```python
from build123d import *

# Parameters (mm, degrees)
SKETCH1_R           = 50.8
BOSS_EXTRUDE1_DEPTH = 228.6
SKETCH2_R           = 63.5
BOSS_EXTRUDE2_DEPTH = 25.4
BOSS_EXTRUDE3_START = 25.4
SKETCH3_R           = 63.5
BOSS_EXTRUDE3_DEPTH = 25.4
CUT_EXTRUDE2_DEPTH  = 12.7
CHAMFER2_SIZE       = 10.16
CHAMFER2_SIZE_2     = 19.940122736
SKETCH5_R           = 38.1
CUT_EXTRUDE5_DEPTH  = 12.7
CHAMFER3_SIZE       = 5.08
CHAMFER3_SIZE2      = 17.716065375
SKETCH6_R           = 31.75
BOSS_EXTRUDE6_DEPTH = 12.7


with BuildPart() as part:
    # Sketch1 → Boss-Extrude1 (new body)
    with BuildSketch(Plane(origin=(0, 0, 0), x_dir=(1, 0, 0), z_dir=(0, 1, 0))):
        with Locations(Location((0, 0, 0), (0, 0, 270))):
            Circle(SKETCH1_R)
    extrude(amount=BOSS_EXTRUDE1_DEPTH)

    # Sketch2 → Boss-Extrude2 (add)
    with BuildSketch(Plane(origin=(0, 228.6, 0), x_dir=(1, 0, 0), z_dir=(0, 1, 0))):
        with Locations(Location((0, 0, 0), (0, 0, 270))):
            Circle(SKETCH2_R)
    extrude(amount=BOSS_EXTRUDE2_DEPTH)

    # Sketch3 → Boss-Extrude3 (add)
    with BuildSketch(Plane.XZ.offset(BOSS_EXTRUDE3_START)):
        with Locations(Location((0, 0, 0), (0, 0, 90))):
            Circle(SKETCH3_R)
    extrude(amount=-BOSS_EXTRUDE3_DEPTH)

    # Sketch4 → Cut-Extrude2 (cut)
    with BuildSketch(Plane(origin=(0, 254, 0), x_dir=(1, 0, 0), z_dir=(0, 1, 0))):
        Polygon((0, 43.994090512), (-38.1, 21.997045256), (-38.1, -21.997045256), (0, -43.994090512), (38.1, -21.997045256), (38.1, 21.997045256), align=None)
    extrude(amount=-CUT_EXTRUDE2_DEPTH, mode=Mode.SUBTRACT)

    # Chamfer2
    # the kernel refuses this chamfer: 19.940122736, 10.16 mm, written as the material it takes off along each edge
    with BuildSketch(Plane(origin=(0, 254, 0), x_dir=(0, 0, 1), z_dir=(-1, 0, 0))) as chamfer2_piece_1:
        Polygon((63.5, -CHAMFER2_SIZE), (63.5 - CHAMFER2_SIZE_2, 0), (63.5, 0), align=None)
    revolve(axis=Axis((0, 254, 0), (0, 1, 0)), mode=Mode.SUBTRACT)

    # Sketch5 → Cut-Extrude5 (cut)
    with BuildSketch(Plane.XZ.offset(25.4)):
        Circle(SKETCH5_R)
        with BuildLine():
            Line((19.049999468, 32.995568191), (0, 43.994090512))
            Line((0, 43.994090512), (-19.04999937, 32.995568248))
            ThreePointArc((-19.04999937, 32.995568248), (5.7e-08, 38.1), (19.049999468, 32.995568191))
        make_face()
        with BuildLine():
            Line((38.1, 21.997045256), (19.049999468, 32.995568191))
            ThreePointArc((19.049999468, 32.995568191), (32.995567731, 19.050000266), (38.1, 0))
            Line((38.1, 0), (38.1, 21.997045256))
        make_face()
        with BuildLine():
            ThreePointArc((-38.1, -1.79e-07), (-32.995567747, 19.050000238), (-19.04999937, 32.995568248))
            Line((-19.04999937, 32.995568248), (-38.1, 21.997045256))
            Line((-38.1, 21.997045256), (-38.1, -1.79e-07))
        make_face()
        with BuildLine():
            ThreePointArc((-19.049999051, -32.995568432), (-32.995567566, -19.050000552), (-38.1, -1.79e-07))
            Line((-38.1, -1.79e-07), (-38.1, -21.997045256))
            Line((-38.1, -21.997045256), (-19.049999051, -32.995568432))
        make_face()
        with BuildLine():
            Line((38.1, -21.997045256), (38.1, 0))
            ThreePointArc((38.1, 0), (32.995567731, -19.050000266), (19.049999468, -32.995568191))
            Line((19.049999468, -32.995568191), (38.1, -21.997045256))
        make_face()
        with BuildLine():
            ThreePointArc((19.049999468, -32.995568191), (2.4e-07, -38.1), (-19.049999051, -32.995568432))
            Line((-19.049999051, -32.995568432), (0, -43.994090512))
            Line((0, -43.994090512), (19.049999468, -32.995568191))
        make_face()
    extrude(amount=-CUT_EXTRUDE5_DEPTH, mode=Mode.SUBTRACT)

    # Chamfer3
    chamfer3_edges = [part.edges().sort_by_distance(p)[0] for p in [
        (0, -25.4, -63.5),
    ]]
    chamfer3_side = [part.faces().sort_by_distance(p)[0] for p in [
        (0, -12.7, -63.5),
    ]]
    chamfer(chamfer3_edges, length=CHAMFER3_SIZE, length2=CHAMFER3_SIZE2, reference=chamfer3_side[0])

    # Sketch6 → Boss-Extrude6 (add)
    with BuildSketch(Plane.XZ.offset(12.7)):
        with Locations(Location((0, 0, 0), (0, 0, 270))):
            Circle(SKETCH6_R)
    extrude(amount=BOSS_EXTRUDE6_DEPTH)


solid = part.part
```
Source: CAD feature listing. Evaluate the final solid. Frame: model axes, mm. A direction names the side the tool comes from. Give positions to 0.01 mm unless a question says otherwise; leave off trailing zeros. Order: outer loops, then holes, each group sorted by start corner. A loop starts at its lowest first (then second) coordinate and runs counter-clockwise, first axis right, second up.
(1) Section query B-B (y = 33). Return the cut outline in (x, z).
(2) Access query for faces 1 (the face through (38.1, 248, 0)), 2 (the face through (0, -12.7, -32)), 3 (the face through (61.99, -10.3, -13.77)). Directions: +Z, -Z, +X, -X, +Y, -Y. A direction counts if a zero-diameter tool reaches every point of the face in a straight line with its end or side. Return the directions, or none.
(3) Section query A-A (z = 0). Return the cut outline in (x, y).
(4) Pull-direction query (Z, two-part tool) for faces 4 (the face through (0, -25.4, 0)), 5 (the face through (2, 253.5, -44.5)), 6 (the face through (-38.1, 248, 0)); classes: +Z half, -Z half, draft (parallel to the pull), parting line (faces both ways), or undercut.
(5) Material intervals for line 1 along Y through (x, z) = (22.5, -24); line 2 along Y through (x, z) = (13.5, -10); line 3 along Y through (x, z) = (-42, -40), sorted ascending.
(6) Contact query for flat-ended pins moving along their axis: P1, Ø12, axis at x = -19.5, y = 136, coming from the -Z side; P2, Ø6.5, axis at y = 245.5, z = 5, coming from the -X side; P3, Ø2, axis at x = 37.5, y = 204, coming from the +Z side. Output: stop coordinate, or through.
(7) Section query C-C (y = 233.5). Return the cut outline in (x, z), plus the area to 3 significant figures.
Outcome:
1. outline: circle Ø101.6 at (0, 0)
2. face 1: +Y
2. face 2: -Y
2. face 3: +Y, -Y
3. outline: (-63.5, -20.32) - (-45.78, -25.4) - (-38.1, -25.4) - (-38.1, -12.7) - (-31.75, -12.7) - (-31.75, -25.4) - (31.75, -25.4) - (31.75, -12.7) - (38.1, -12.7) - (38.1, -25.4) - (45.78, -25.4) - (63.5, -20.32) - (63.5, 0) - (50.8, 0) - (50.8, 228.6) - (63.5, 228.6) - (63.5, 243.84) - (43.56, 254) - (38.1, 254) - (38.1, 241.3) - (-38.1, 241.3) - (-38.1, 254) - (-43.56, 254) - (-63.5, 243.84) - (-63.5, 228.6) - (-50.8, 228.6) - (-50.8, 0) - (-63.5, 0) - close
4. face 4: draft
4. face 5: parting line
4. face 6: undercut
5. line 1: y = -12.7 to 241.3
5. line 2: y = -25.4 to 241.3
5. line 3: y = -21.9 to 0, 228.6 to 246.64
6. P1: stops at z = -48.97
6. P2: stops at x = -63.46
6. P3: stops at z = 35.33
7. outline: circle Ø127 at (0, 0)
7. area: 12,700 mm2
